```python
from build123d import *

# Parameters (mm, degrees)
SKETCH1_W                          = 152.4
SKETCH1_H                          = 152.4
EXTRUDE1_DEPTH                     = 6.35
F_3_4_0_75_DIAMETER_HOLE1_D        = 19.05
F_3_4_0_75_DIAMETER_HOLE1_DEPTH    = 112.776
F_3_4_0_75_DIAMETER_HOLE1_TIP      = 5.723197396
EXTRUDE_THIN1_DEPTH                = 88.9
F_9_16_0_5625_DIAMETER_HOLE1_D     = 14.2875
F_9_16_0_5625_DIAMETER_HOLE1_DEPTH = 112.776
F_9_16_0_5625_DIAMETER_HOLE1_TIP   = 4.292398047


with BuildPart() as part:
    # Sketch1 → Extrude1 (new body)
    with BuildSketch(Plane(origin=(0, 0, 0), x_dir=(1, 0, 0), z_dir=(0, 1, 0))):
        Rectangle(SKETCH1_W, SKETCH1_H)
    extrude(amount=EXTRUDE1_DEPTH)

    # 3/4 (0.75) Diameter Hole1
    with Locations(Plane(origin=(0, 6.35, 0), x_dir=(-1, 0, 0), z_dir=(0, 1, 0))):
        with Locations((53.975, -53.975), (-53.975, -53.975), (-53.975, 53.975), (53.975, 53.975)):
            Hole(F_3_4_0_75_DIAMETER_HOLE1_D / 2, depth=F_3_4_0_75_DIAMETER_HOLE1_DEPTH)
            with Locations((0, 0, -(F_3_4_0_75_DIAMETER_HOLE1_DEPTH + F_3_4_0_75_DIAMETER_HOLE1_TIP / 2))):  # 118° drill point
                Cone(0, F_3_4_0_75_DIAMETER_HOLE1_D / 2, F_3_4_0_75_DIAMETER_HOLE1_TIP, mode=Mode.SUBTRACT)

    # Sketch4 → Extrude-Thin1 (add)
    with BuildSketch(Plane(origin=(0, 6.35, 0), x_dir=(1, 0, 0), z_dir=(0, 1, 0))):
        with BuildLine():
            Line((-20.955, 19.685), (-20.955, -19.685))
            ThreePointArc((-20.955, -19.685), (-20.211051224, -21.481051224), (-18.415, -22.225))
            Line((-18.415, -22.225), (18.415, -22.225))
            ThreePointArc((18.415, -22.225), (20.211051224, -21.481051224), (20.955, -19.685))
            Line((20.955, -19.685), (20.955, 19.685))
            Line((20.955, 19.685), (23.6474, 19.685))
            Line((23.6474, 19.685), (23.6474, -19.685))
            ThreePointArc((23.6474, -19.685), (22.114865522, -23.384865522), (18.415, -24.9174))
            Line((18.415, -24.9174), (-18.415, -24.9174))
            ThreePointArc((-18.415, -24.9174), (-22.114865522, -23.384865522), (-23.6474, -19.685))
            Line((-23.6474, -19.685), (-23.6474, 19.685))
            Line((-23.6474, 19.685), (-20.955, 19.685))
        make_face()
    extrude(amount=EXTRUDE_THIN1_DEPTH)

    # 9/16 (0.5625) Diameter Hole1
    with Locations(Plane(origin=(23.6474, 0, 0), x_dir=(0, 0, -1), z_dir=(1, 0, 0))):
        with Locations((0, 73.025), (0, 28.575)):
            Hole(F_9_16_0_5625_DIAMETER_HOLE1_D / 2, depth=F_9_16_0_5625_DIAMETER_HOLE1_DEPTH)
            with Locations((0, 0, -(F_9_16_0_5625_DIAMETER_HOLE1_DEPTH + F_9_16_0_5625_DIAMETER_HOLE1_TIP / 2))):  # 118° drill point
                Cone(0, F_9_16_0_5625_DIAMETER_HOLE1_D / 2, F_9_16_0_5625_DIAMETER_HOLE1_TIP, mode=Mode.SUBTRACT)


solid = part.part
```
Source: CAD feature listing. Evaluate the final solid. Frame: model axes, mm. A direction names the side the tool comes from. Round coordinates to 2 decimals unless told otherwise and drop trailing zeros. Loops run counter-clockwise (first coordinate to the right, second up) from the corner with the lowest first, then second, coordinate; pieces in that order, holes last.
(1) Section query B-B (x = -52.5). Output: boundary loops of the cut face in (y, z), and give its area (3 significant figures).
From the geometry:
outline: (0, -76.2) - (6.35, -76.2) - (6.35, -63.39) - (0, -63.39) - close; (0, -44.56) - (6.35, -44.56) - (6.35, 44.56) - (0, 44.56) - close; (0, 63.39) - (6.35, 63.39) - (6.35, 76.2) - (0, 76.2) - close
area: 729 mm2
(2) Contact query for flat-ended pins moving along their axis: pin 1 Ø23 at (y, z) = (28.575, 0) entering from +X; pin 2 Ø2 at (x, y) = (22.5, 44.5) entering from -Z (3 decimals); pin 3 Ø1 at (x, z) = (16.5, -58.5) entering from +Y. Output: stop coordinate, or through.
From the geometry:
pin 1: stops at x = 23.65
pin 2: stops at z = -19.685
pin 3: stops at y = 6.35
(3) Section query A-A (z = 0). Output: boundary loops of the cut face in (x, y) (3 decimals).
From the geometry:
outline: (-76.2, 0) - (76.2, 0) - (76.2, 6.35) - (23.647, 6.35) - (23.647, 21.431) - (20.955, 21.431) - (20.955, 6.35) - (-20.955, 6.35) - (-20.955, 21.431) - (-23.647, 21.431) - (-23.647, 6.35) - (-76.2, 6.35) - close; (-23.647, 35.719) - (-20.955, 35.719) - (-20.955, 65.881) - (-23.647, 65.881) - close; (-23.647, 80.169) - (-20.955, 80.169) - (-20.955, 95.25) - (-23.647, 95.25) - close; (20.955, 35.719) - (23.647, 35.719) - (23.647, 65.881) - (20.955, 65.881) - close; (20.955, 80.169) - (23.647, 80.169) - (23.647, 95.25) - (20.955, 95.25) - close
(4) Pull-direction query (Y, two-part tool) for faces 6 (the cylindrical face through (22.28, 21.6, -1.55)), 7 (the cylindrical face through (-61.534, 3.131, -59.771)), 8 (the flat face through (4, 95.25, 24)); classes: +Y half, -Y half, draft (parallel to the pull), parting line (faces both ways), or undercut.
From the geometry:
face 6: undercut
face 7: draft
face 8: +Y half
(5) Material intervals for probe 1 along Y at (x, z) = (-22.5, 0); probe 2 along X at (y, z) = (14, 6.5) (3 decimals); probe 3 along X at (y, z) = (4.5, -52), sorted ascending.
From the geometry:
probe 1: y = 0 to 21.43, 35.72 to 65.88, 80.17 to 95.25
probe 2: x = -23.647 to -20.955, 20.955 to 23.647
probe 3: x = -76.2 to -63.29, -44.66 to 44.66, 63.29 to 76.2
(6) Section query D-D (z = 60.5). Output: boundary loops of the cut face in (x, y), and give its area (3 significant figures).
From the geometry:
outline: (-76.2, 0) - (-60.91, 0) - (-60.91, 6.35) - (-76.2, 6.35) - close; (-47.04, 0) - (47.04, 0) - (47.04, 6.35) - (-47.04, 6.35) - close; (60.91, 0) - (76.2, 0) - (76.2, 6.35) - (60.91, 6.35) - close
area: 791 mm2
(7) Access query for faces 1 (the cylindrical face through (22.2, 50.2, 23.3)), 2 (the cylindrical face through (-22.1, 50.2, 23.4)), 3 (the flat face through (-23.647, 50, 0)), 4 (the cylindrical face through (-22.32, 21.6, -1.55)), 5 (the flat face through (0, 50, 22.225)). Directions: +Z, -Z, +X, -X, +Y, -Y. A direction counts if a zero-diameter tool reaches every point of the face in a straight line with its end or side. Return the directions, or none.
From the geometry:
face 1: +Z, +X, +Y
face 2: +Z, -X, +Y
face 3: +Z, -Z, -X, +Y
face 4: +X, -X
face 5: -Z, +Y
(8) Section query C-C (y = 12.5). Output: boundary loops of the cut face in (x, z) (3 decimals).
From the geometry:
outline: (-23.647, -19.685) - (-20.955, -19.685) - (-20.955, 19.685) arc R2.54 cw to (-18.415, 22.225) - (18.415, 22.225) arc R2.54 cw to (20.955, 19.685) - (20.955, -19.685) - (23.647, -19.685) - (23.647, 19.685) arc R5.232 ccw to (18.415, 24.917) - (-18.415, 24.917) arc R5.232 ccw to (-23.647, 19.685) - close
